Autodesk Inventor part; units mm, degrees
ref_plane "YZ Plane" through (0, 0, 0) normal (1, 0, 0) x (0, 1, 0)
ref_plane "XZ Plane" through (0, 0, 0) normal (0, 1, 0) x (-1, 0, 0)
ref_plane "XY Plane" through (0, 0, 0) normal (0, 0, 1) x (1, 0, 0)
sketch "Эскиз3" plane through (0, 0, 0) normal (0, 0, 1) x (1, 0, 0)
  circle A0 centre (0, 0) radius 10
  arc A1 (22.3607, 20) -> (22.3607, -20) centre (0, 0) ccw
  line L0 (22.3607, 20) -> (100, 20)
  line L1 (100, 20) -> (100, -20)
  line L2 (100, -20) -> (22.3607, -20)
  line L3 (22.3607, -20) -> (22.3607, 20)
  dimension "d8" = 20
  dimension "d9" = 60
  dimension "d10" = 100
  dimension "d11" = 40
extrude "Выдавливание3" add sketch "Эскиз3" along normal blind 3
equation "\"d8\" = d_main_shaft"
equation "\"d11\" = hight_coxa"
equation "\"d6\" = thickness_steel"
equation "\"tolerance_plazma\" = 0.1"
equation "\"thickness_steel\" = 3"
equation "\"d_main_screw_holes\" = 6.1"
equation "\"d_main_shaft\" = 20"
equation "\"thickness_profile_tibea\" = 3"
equation "\"hight_shaft_shift\" = 37"
equation "\"thickness_profile_femur\" = 3"
equation "\"width_shaft_shift\" = 35"
equation "\"width_flattened_surface\" = 12"
equation "\"length_coxa\" = 100"
equation "\"hight_coxa\" = 40"
properties part number "coxa_support_steel" material "Сталь"
Geometry: final body of the model. Coordinates: model frame, mm. A direction names the side the tool comes from. Coordinates: 2 decimals unless noted, no trailing zeros. Order: outer loops, then holes, each group sorted by start corner. A loop starts at its lowest first (then second) coordinate and runs counter-clockwise, first axis right, second up.
Item 1: Contact query for flat-ended pins moving along their axis: P1, Ø1.5, axis at x = 48, z = 1.5, coming from the +Y side; P2, Ø1.5, axis at x = 52, z = 1, coming from the -Y side; P3, Ø16, axis at x = 0, y = 0, coming from the +Z side. Output: stop coordinate, or through.
Answer:
P1: stops at y = 20
P2: stops at y = -20
P3: passes through
Item 2: Access query for faces 1 (the face through (34, 0, 0)), 2 (the face through (61, 20, 1)). Directions: +Z, -Z, +X, -X, +Y, -Y. A direction counts if a zero-diameter tool reaches every point of the face in a straight line with its end or side. Return the directions, or none.
Answer:
face 1: -Z, +X, -X, +Y, -Y
face 2: +Z, -Z, +X, +Y
Item 3: Section query A-A (y = 0). Output: boundary loops of the cut face in (x, z), then the cut area to 3 significant figures.
Answer:
outline: (-30, 0) - (-10, 0) - (-10, 3) - (-30, 3) - close; (10, 0) - (100, 0) - (100, 3) - (10, 3) - close
area: 330 mm2
Item 4: Section query C-C (z = 2.25). Output: boundary loops of the cut face in (x, y), then the cut area to 3 significant figures.
Answer:
outline: (22.36, -20) - (100, -20) - (100, 20) - (22.36, 20) arc R30 ccw (long way) to start; hole circle Ø20 at (0, 0)
area: 5,410 mm2
Item 5: Section query D-D (x = 39.5). Output: boundary loops of the cut face in (y, z), then the cut area to 3 significant figures.
Answer:
outline: (-20, 0) - (20, 0) - (20, 3) - (-20, 3) - close
area: 120 mm2
Item 6: Material intervals for line 1 along Y through (x, z) = (0, 0.85); line 2 along Y through (x, z) = (29, 1.75); line 3 along X through (y, z) = (6.5, 1.4), sorted ascending.
Answer:
line 1: y = -30 to -10, 10 to 30
line 2: y = -20 to 20
line 3: x = -29.29 to -7.6, 7.6 to 100
Item 7: Section query B-B (x = 0). Output: boundary loops of the cut face in (y, z), then the cut area to 3 significant figures.
Answer:
outline: (-30, 0) - (-10, 0) - (-10, 3) - (-30, 3) - close; (10, 0) - (30, 0) - (30, 3) - (10, 3) - close
area: 120 mm2
Item 8: Draft query along Y for faces 3 (the face through (100, 0, 1)), 4 (the face through (-29.983, -1.013, 1.479)), 5 (the face through (-2.17, 9.76, 1.48)), 6 (the face through (62, -20, 1)). Return one class per face: released by +Y, released by -Y, zero draft, split by the parting line, or undercut.
Answer:
face 3: zero draft
face 4: split by the parting line
face 5: undercut
face 6: released by -Y
